The listing builds one solid part. Answer for the finished solid, in the listing's coordinates (mm). A direction names the side the tool comes from. Coordinates: 2 decimals unless noted, no trailing zeros. Write each loop counter-clockwise with the first axis right and the second up, starting at its lowest first coordinate (ties: lowest second). Pieces come first, ordered by that corner, then holes.
Autodesk Inventor part; units mm, degrees
ref_plane "Work Plane1" through (-19.25, -0.5, 9.85) normal (0, 0, 1) x (1, 0, 0)
ref_plane "Work Plane2" through (-19.25, -0.5, 12.85) normal (0, 0, 1) x (1, 0, 0)
ref_plane "Work Plane4" through (19.95, -28.3, 9.85) normal (1, 0, 0) x (0, 0, -1)
ref_plane "Work Plane1" through (-19.25, -0.5, 9.85) normal (0, 0, 1) x (1, 0, 0)
sketch "Sketch1" plane through (-19.25, -0.5, 9.85) normal (0, 0, 1) x (1, 0, 0)
  line L0 (-0.695, -27.8) -> (39.2, -27.8)
  line L1 (39.2, -27.8) -> (39.2, 8.9608)
  line L2 (39.2, 8.9608) -> (-0.695, 8.9608)
  line L3 (-0.695, 8.9608) -> (-0.695, -27.8)
  point P0 (19.25, 0.5)
extrude "Extrusion1" add sketch "Sketch1" along normal blind 3
ref_plane "Work Plane2" through (-19.25, -0.5, 12.85) normal (0, 0, 1) x (1, 0, 0)
sketch "Sketch2" plane through (-19.25, -0.5, 12.85) normal (0, 0, 1) x (1, 0, 0)
  line L0 (39.2, -27.8) -> (39.2, 8.9608)
  line L1 (39.2, -27.8) -> (-0.695, -27.8)
  line L2 (-0.695, -27.8) -> (-0.695, 8.9608)
  line L3 (-0.695, 8.9608) -> (39.2, 8.9608)
  line L4 (39.2, 8.9608) -> (39.2, -27.8)
  point P0 (19.25, 0.5)
  point P1 (39.2, 8.9608)
extrude "Extrusion2" add sketch "Sketch2" along normal blind 5
ref_plane "Work Plane4" through (19.95, -28.3, 9.85) normal (1, 0, 0) x (0, 0, -1)
sketch "Sketch3" plane through (19.95, -28.3, 9.85) normal (1, 0, 0) x (0, 0, -1)
  line L0 (0, 0) -> (0, 36.7608)
  line L1 (0, 0) -> (-8, 0)
  line L2 (0, 36.7608) -> (-2, 36.7608)
  line L3 (-2, 36.7608) -> (-2, 0)
  line L4 (-2, 0) -> (0, 0)
  line L5 (0, 0) -> (0, 36.7608)
  point P0 (9.85, 28.3)
  dimension "d4" = 2
extrude "Extrusion3" cut sketch "Sketch3" against normal blind 50
ref_plane "Work Plane3" through (19.95, -28.3, 17.85) normal (1, 0, 0) x (0, 0, -1)
sketch "Sketch4" plane through (19.95, -28.3, 17.85) normal (1, 0, 0) x (0, 0, -1)
  line L0 (6, 0) -> (0, 0)
  line L1 (6, 36.7608) -> (0, 36.7608)
  line L2 (0, 0) -> (1, 0)
  line L3 (1, 0) -> (1, 36.7608)
  line L4 (1, 36.7608) -> (0, 36.7608)
  line L5 (0, 36.7608) -> (0, 0)
  point P0 (17.85, 28.3)
  point P1 (1, 0)
  dimension "d7" = 1
extrude "Extrusion4" cut sketch "Sketch4" against normal blind 50
ref_plane "Work Plane5" through (19.95, -28.3, 11.85) normal (1, 0, 0) x (0, 0, -1)
sketch "Sketch5" plane through (19.95, -28.3, 11.85) normal (1, 0, 0) x (0, 0, -1)
  line L0 (-5, 36.7608) -> (-5, 0)
  line L1 (0, 0) -> (0, 36.7608)
  line L2 (-5, 36.7608) -> (0, 36.7608)
  line L3 (0, 36.7608) -> (0, 0)
  line L4 (0, 0) -> (-5, 0)
  line L5 (-5, 0) -> (-5, 36.7608)
  point P0 (11.85, 28.3)
extrude "Extrusion5" add sketch "Sketch5" along normal blind 7
ref_plane "Work Plane6" through (-19.945, -28.3, 11.85) normal (0, 0, -1) x (-1, 0, 0)
sketch "Sketch6" plane through (-19.945, -28.3, 11.85) normal (0, 0, -1) x (-1, 0, 0)
  line L0 (-46.895, 0) -> (-46.895, 36.7608)
  line L1 (-46.895, 27.8459) -> (-40.895, 27.8459)
  line L2 (-40.895, 27.8459) -> (-40.895, 11.8459)
  line L3 (-40.895, 11.8459) -> (-46.895, 11.8459)
  line L4 (-46.895, 11.8459) -> (-46.895, 27.8459)
  point P0 (-19.945, 28.3)
  dimension "d12" = 6
  dimension "d13" = 16
extrude "Extrusion6" add sketch "Sketch6" along normal blind 22.875
sketch "Sketch7" plane through (20.95, -0.4541, 11.85) normal (0, 1, 0) x (1, 0, 0)
  arc A0 (5.4164, 8.2173) -> (5.4164, 5.6327) centre (3.7611, 6.925) ccw
  circle A1 centre (3.7611, 6.925) radius 2.5
  arc A2 (5.4164, 18.0673) -> (5.4164, 15.4827) centre (3.7611, 16.775) ccw
  circle A3 centre (3.7611, 16.775) radius 2.5
  point P0 (-20.95, 11.85)
  dimension "d16" = 5
  dimension "d17" = 5
extrude "Extrusion7" cut sketch "Sketch7" against normal blind 22.875
ref_plane "Work Plane7" through (26.95, -28.3, 11.85) normal (1, 0, 0) x (0, 0, -1)
sketch "Sketch8" plane through (26.95, -28.3, 11.85) normal (1, 0, 0) x (0, 0, -1)
  line L0 (0, 11.8459) -> (22.875, 11.8459)
  line L1 (22.875, 27.8459) -> (22.875, 11.8459)
  line L2 (0, 11.8459) -> (22.875, 11.8459)
  line L3 (22.875, 11.8459) -> (22.875, 16.8459)
  line L4 (22.875, 16.8459) -> (0, 16.8459)
  line L5 (0, 16.8459) -> (0, 11.8459)
  point P0 (11.85, 28.3)
  dimension "d20" = 5
extrude "Extrusion8" cut sketch "Sketch8" against normal blind 6.7
ref_plane "Work Plane8" through (-19.945, -28.3, 11.85) normal (-1, 0, 0) x (0, 0, 1)
sketch "Sketch9" plane through (-19.945, -28.3, 11.85) normal (-1, 0, 0) x (0, 0, 1)
  line L0 (0, 36.7608) -> (0, 0)
  line L1 (5, 0) -> (0, 0)
  line L2 (0, 36.7608) -> (5, 36.7608)
  line L3 (5, 36.7608) -> (5, 0)
  line L4 (5, 0) -> (0, 0)
  line L5 (0, 0) -> (0, 36.7608)
  point P0 (-11.85, 28.3)
extrude "Extrusion9" add sketch "Sketch9" along normal blind 7
ref_plane "Work Plane10" through (26.95, -0.4541, 11.85) normal (0, 0, -1) x (-1, 0, 0)
sketch "Sketch11" plane through (26.95, -0.4541, 11.85) normal (0, 0, -1) x (-1, 0, 0)
  line L0 (53.895, -27.8459) -> (53.895, 8.9148)
  line L1 (53.895, 0) -> (47.895, 0)
  line L2 (47.895, 0) -> (47.895, -11)
  line L3 (47.895, -11) -> (53.895, -11)
  line L4 (53.895, -11) -> (53.895, 0)
  point P0 (26.95, 0.4541)
  dimension "d25" = 6
extrude "Extrusion10" add sketch "Sketch11" along normal blind 22.875
sketch "Sketch12" plane through (-26.945, -0.4541, 11.85) normal (0, 1, 0) x (1, 0, 0)
  arc A0 (0.5786, 15.4827) -> (0.5786, 18.0673) centre (2.2339, 16.775) ccw
  circle A1 centre (2.2339, 16.775) radius 2.5
  arc A2 (0.5786, 5.6327) -> (0.5786, 8.2173) centre (2.2339, 6.925) ccw
  circle A3 centre (2.2339, 6.925) radius 2.5
  point P0 (26.945, 11.85)
  dimension "d28" = 5
  dimension "d29" = 5
extrude "Extrusion11" cut sketch "Sketch12" against normal blind 22.875
ref_plane "Work Plane11" through (-26.945, -28.3, 11.85) normal (-1, 0, 0) x (0, 0, 1)
sketch "Sketch13" plane through (-26.945, -28.3, 11.85) normal (-1, 0, 0) x (0, 0, 1)
  line L0 (0, 16.8459) -> (0, 27.8459)
  line L1 (5, 36.7608) -> (0, 36.7608)
  line L2 (0, 27.8459) -> (5, 27.8459)
  line L3 (5, 27.8459) -> (5, 36.7608)
  line L4 (5, 36.7608) -> (0, 36.7608)
  line L5 (0, 36.7608) -> (0, 27.8459)
  point P0 (-11.85, 28.3)
extrude "Extrusion12" cut sketch "Sketch13" against normal blind 67.325
ref_plane "Work Plane9" through (26.95, -28.3, 11.85) normal (0, -1, 0) x (1, 0, 0)
sketch "Sketch14" plane through (26.95, -28.3, 11.85) normal (0, -1, 0) x (1, 0, 0)
  line L0 (0, 5) -> (0, 0)
  line L1 (0, 5) -> (-53.895, 5)
  line L2 (0, 0) -> (-53.895, 0)
  line L3 (-53.895, 0) -> (-53.895, 5)
  line L4 (-53.895, 5) -> (0, 5)
  line L5 (0, 5) -> (0, 0)
  point P0 (-26.95, -11.85)
extrude "Extrusion13" add sketch "Sketch14" along normal blind 5
ref_plane "Work Plane12" through (26.95, -11.4541, 11.85) normal (0, 0, -1) x (-1, 0, 0)
sketch "Sketch15" plane through (26.95, -11.4541, 11.85) normal (0, 0, -1) x (-1, 0, 0)
  line L0 (53.895, -21.8459) -> (0, -21.8459)
  line L1 (53.895, 11) -> (53.895, -21.8459)
  line L2 (0, -21.8459) -> (53.895, -21.8459)
  line L3 (53.895, -21.8459) -> (53.895, -17.8459)
  line L4 (53.895, -17.8459) -> (0, -17.8459)
  line L5 (0, -17.8459) -> (0, -21.8459)
  point P0 (26.95, 11.4541)
  dimension "d36" = 4
extrude "Extrusion14" add sketch "Sketch15" along normal blind 22.4625
ref_plane "Work Plane13" through (-26.945, -29.3, 11.85) normal (0, 1, 0) x (1, 0, 0)
sketch "Sketch16" plane through (-26.945, -29.3, 11.85) normal (0, 1, 0) x (1, 0, 0)
  line L0 (53.895, 0) -> (53.895, 22.4625)
  line L1 (0, 0) -> (0, 22.4625)
  line L2 (53.895, 0) -> (0, 0)
  line L3 (0, 0) -> (0, 1)
  line L4 (0, 1) -> (53.895, 1)
  line L5 (53.895, 1) -> (53.895, 0)
  point P0 (26.945, 11.85)
  point P1 (53.895, 1)
  dimension "d39" = 1
extrude "Extrusion15" add sketch "Sketch16" along normal blind 30
ref_plane "Work Plane14" through (26.95, -28.3, 11.85) normal (1, 0, 0) x (0, 0, -1)
sketch "Sketch17" plane through (26.95, -28.3, 11.85) normal (1, 0, 0) x (0, 0, -1)
  line L0 (0, 29) -> (1, 29)
  line L1 (5.8126, 27.8459) -> (1, 27.8459)
  line L2 (0, 29) -> (1, 29)
  line L3 (1, 29) -> (1, 27.8459)
  line L4 (1, 27.8459) -> (0, 27.8459)
  line L5 (0, 27.8459) -> (0, 29)
  point P0 (11.85, 28.3)
extrude "Extrusion16" cut sketch "Sketch17" against normal blind 100
sketch "Sketch19" plane through (26.95, -33.3, 11.85) normal (0, -1, 0) x (1, 0, 0)
  circle A0 centre (-16.85, -11.85) radius 5
  circle A1 centre (-16.85, -11.85) radius 1.5
  point P0 (-26.95, -11.85)
  dimension "d47" = 10
  dimension "d50" = 3
extrude "Extrusion20" cut sketch "Sketch19" against normal blind 10 contours A1
sketch "Sketch20" plane through (26.95, -33.3, 11.85) normal (0, -1, 0) x (1, 0, 0)
  line L0 (-53.895, -22.4625) -> (0, -22.4625)
  line L1 (-53.895, 5) -> (-53.895, -22.4625)
  line L2 (0, -22.4625) -> (-53.895, -22.4625)
  line L3 (-53.895, -22.4625) -> (-53.895, 5)
  line L4 (-53.895, 5) -> (0, 5)
  line L5 (0, 5) -> (0, -22.4625)
  point P0 (-26.95, -11.85)
extrude "Extrusion21" add sketch "Sketch20" along normal blind 2
sketch "Sketch21" plane through (-26.945, -29.3, -10.6125) normal (0, 1, 0) x (1, 0, 0)
  circle A0 centre (37.045, -10.6125) radius 1.5
  circle A1 centre (37.045, -10.6125) radius 1.5
  point P0 (26.945, -10.6125)
extrude "Extrusion22" cut sketch "Sketch21" against normal blind 10
sketch "Sketch22" plane through (-26.945, -29.3, -10.6125) normal (0, 1, 0) x (1, 0, 0)
  circle A0 centre (37.045, -10.6125) radius 1.5
  circle A1 centre (37.045, -10.6125) radius 2.5
  point P0 (26.945, -10.6125)
  dimension "d59" = 5
extrude "Extrusion23" cut sketch "Sketch22" against normal blind 2
sketch "Sketch23" plane through (-19.945, -28.3, -11.025) normal (0, 0, -1) x (-1, 0, 0)
  line L0 (-46.895, 27.8459) -> (-46.895, 16.8459)
  line L1 (-46.895, 27.8459) -> (-48.895, 27.8459)
  line L2 (-48.895, 27.8459) -> (-48.895, 16.8459)
  line L3 (-48.895, 16.8459) -> (-46.895, 16.8459)
  line L4 (-46.895, 16.8459) -> (-46.895, 27.8459)
  line L5 (7, 16.8459) -> (7, 27.8459)
  line L6 (7, 27.8459) -> (9, 27.8459)
  line L7 (9, 27.8459) -> (9, 16.8459)
  line L8 (9, 16.8459) -> (7, 16.8459)
  line L9 (7, 16.8459) -> (7, 27.8459)
  point P0 (-19.945, 28.3)
  dimension "d62" = 2
  dimension "d63" = 2
extrude "Extrusion24" add sketch "Sketch23" against normal up to surface (27.875 mm away)
sketch "Sketch24" plane through (-20.945, -0.4541, 10.85) normal (0, 1, 0) x (1, 0, 0)
  arc A0 (47.895, 7.0374) -> (47.895, 4.8126) centre (45.6561, 5.925) ccw
  circle A1 centre (45.6561, 5.925) radius 1.6
  arc A2 (47.895, 16.8874) -> (47.895, 14.6626) centre (45.6561, 15.775) ccw
  circle A3 centre (45.6561, 15.775) radius 1.6
  circle A4 centre (45.6561, 5.925) radius 2.5
  circle A5 centre (45.6561, 15.775) radius 2.5
  point P0 (20.945, 10.85)
  point P1 (47.895, 4.8126)
  dimension "d66" = 3.2
  dimension "d67" = 3.2
extrude "Extrusion25" add sketch "Sketch24" against normal up to surface (11 mm away)
sketch "Sketch25" plane through (-20.945, -0.4541, 10.85) normal (0, 1, 0) x (1, 0, 0)
  arc A0 (-6, 4.8025) -> (-6, 7.0475) centre (-3.7661, 5.925) ccw
  circle A1 centre (-3.7661, 5.925) radius 1.6
  arc A2 (-6, 14.6525) -> (-6, 16.8975) centre (-3.7661, 15.775) ccw
  circle A3 centre (-3.7661, 15.775) radius 1.6
  circle A4 centre (-3.7661, 15.775) radius 2.5
  circle A5 centre (-3.7661, 5.925) radius 2.5
  point P0 (20.945, 10.85)
  point P1 (-6, 7.0475)
  dimension "d70" = 3.2
  dimension "d71" = 3.2
  dimension "d72" = 5
  dimension "d73" = 5
extrude "Extrusion26" add sketch "Sketch25" against normal up to surface (11 mm away)
sketch "Sketch26" plane through (-26.945, -35.3, 16.85) normal (0, 0, 1) x (1, 0, 0)
  line L0 (55.895, 34.8459) -> (-2, 34.8459)
  line L1 (53.895, 23.8459) -> (55.895, 23.8459)
  line L2 (-2, 34.8459) -> (55.895, 34.8459)
  line L3 (55.895, 34.8459) -> (55.895, 23.8459)
  line L4 (55.895, 23.8459) -> (-2, 23.8459)
  line L5 (-2, 23.8459) -> (-2, 34.8459)
  point P0 (26.945, 35.3)
extrude "Extrusion27" add sketch "Sketch26" along normal blind 20
sketch "Sketch27" plane through (-20.945, -0.4541, 10.85) normal (0, 1, 0) x (1, 0, 0)
  line L0 (49.895, 21.875) -> (49.895, -26)
  line L1 (49.895, -26) -> (49.895, -16)
  line L2 (49.895, -16) -> (-8, -16)
  line L3 (-8, 21.875) -> (-8, -26)
  line L4 (49.895, -16) -> (31.895, -16)
  line L5 (-8, -16) -> (10, -16)
  circle A0 centre (31.895, -16) radius 5
  circle A1 centre (10, -16) radius 5
  point P0 (20.945, 10.85)
  dimension "d78" = 10
  dimension "d79" = 18
  dimension "d80" = 18
  dimension "d81" = 10
  dimension "d82" = 10
hole "Hole1" at (-10.945, -0.4541, 26.85) at (10.95, -0.4541, 26.85) direction (0, -1, 0) diameter 5 end through all countersink diameter 10 countersink angle 90
sketch "Sketch28" plane through (-26.945, -29.3, -10.6125) normal (0, 1, 0) x (1, 0, 0)
  circle A0 centre (37.045, -10.6125) radius 2.5
  line L0 (37.045, -10.6125) -> (53.895, -10.6125)
  line L1 (53.895, 0) -> (53.895, -27.4625)
  line L2 (0, -27.4625) -> (0, 0)
  line L3 (0, -10.6125) -> (16.85, -10.6125)
  line L4 (0, -10.6125) -> (16.85, -10.6125) construction
  line L5 (16.85, -10.6125) -> (37.045, -10.6125)
  circle A1 centre (16.85, -10.6125) radius 1.5
  point P0 (26.945, -10.6125)
  dimension "d90" = 16.85
  dimension "d91" = 0
  dimension "d92" = 3
extrude "Extrusion28" cut sketch "Sketch28" against normal blind 10 contours A1 L3 L5 | L5 L3 A1
sketch "Sketch29" plane through (-26.945, -29.3, -10.6125) normal (0, 1, 0) x (1, 0, 0)
  circle A0 centre (16.85, -10.6125) radius 1.5
  circle A1 centre (16.85, -10.6125) radius 2.5
  point P0 (26.945, -10.6125)
  dimension "d95" = 5
extrude "Extrusion29" cut sketch "Sketch29" against normal up to surface (2 mm away) contours A0 | A1
sketch "Sketch30" plane through (-26.945, -29.3, -10.6125) normal (0, 1, 0) x (1, 0, 0)
  circle A0 centre (37.045, -10.6125) radius 2.5
  circle A1 centre (37.045, -10.6125) radius 2.5
  point P0 (26.945, -10.6125)
extrude "Extrusion30" add sketch "Sketch30" against normal up to surface (6 mm away)
properties part number "woodHold" material "钢"
Q1. Determine the mould class of faces 4 (the face through (-11.594, -33.272, -0.066)), 5 (the face through (0, -6, 36.85)), 6 (the face through (26.95, -31, 9)) for opening direction X: released by +X, released by -X, zero draft, split by the parting line, or undercut.
Answers below:
face 4: undercut
face 5: zero draft
face 6: released by +X
Q2. Given pin 1 (1.8 mm diameter, centred on x = -10.095, z = 0, fed in from +Y); pin 2 (1 mm diameter, centred on x = 1, y = -28.5, fed in from +Z); pin 3 (1.5 mm diameter, centred on x = -11, z = 0, fed in from +Y); pin 4 (14.5 mm diameter, centred on x = 4.5, y = -16, fed in from -Z), each flat-ended and moving along its own axis, determine where each tip first touches the part or whether it passes through.
Answers below:
pin 1: passes through
pin 2: stops at z = 16.85
pin 3: stops at y = -31.3
pin 4: stops at z = 10.85
Q3. The part is cut by section A-A, the plane z = 0. Write down the section's boundary in (x, y) (3 decimals).
Answers below:
outline: (-28.945, -11.454) - (-20.945, -11.454) - (-20.945, -0.454) - (-28.945, -0.454) - close; (-26.945, -35.3) - (-11.595, -35.3) - (-11.595, -31.3) - (-12.595, -31.3) - (-12.595, -29.3) - (-26.945, -29.3) - close; (-8.595, -35.3) - (26.95, -35.3) - (26.95, -29.3) - (-7.595, -29.3) - (-7.595, -31.3) - (-8.595, -31.3) - close; (20.95, -11.454) - (28.95, -11.454) - (28.95, -0.454) - (20.95, -0.454) - close
Q4. Which of the six approach directions +Z, -Z, +X, -X, +Y, -Y give full straight-line access (tool end or side, diameter ignored) to faces 1 (the face through (0, -29.3, 0)), 2 (the face through (0, -23, 16.85)), 3 (the face through (23.532, -5.877, 3.844))?
Answers below:
face 1: -Z, +X, -X
face 2: +Z, +X, -X, -Y
face 3: +Y
Q5. The part is cut by section D-D, the plane x = 1. Write down the section's boundary in (y, z), then the cut area to 3 significant figures.
Answers below:
outline: (-35.3, -10.61) - (-29.3, -10.61) - (-29.3, 10.85) - (-0.45, 10.85) - (-0.45, 36.85) - (-11.45, 36.85) - (-11.45, 16.85) - (-35.3, 16.85) - close
area: 558 mm2
Q6. The part is cut by section C-C, the plane z = 26.85. Write down the section's boundary in (x, y) (3 decimals), then the cut area to 3 significant figures.
Answers below:
outline: (-28.945, -11.454) - (-13.445, -11.454) - (-13.445, -2.954) - (-15.945, -0.454) - (-28.945, -0.454) - close; (-8.445, -11.454) - (8.45, -11.454) - (8.45, -2.954) - (5.95, -0.454) - (-5.945, -0.454) - (-8.445, -2.954) - close; (13.45, -11.454) - (28.95, -11.454) - (28.95, -0.454) - (15.95, -0.454) - (13.45, -2.954) - close
area: 514 mm2
Q7. The part is cut by section B-B, the plane x = 10.95. Write down the section's boundary in (y, z), then the cut area to 3 significant figures.
Answers below:
outline: (-35.3, -10.61) - (-29.3, -10.61) - (-29.3, 10.85) - (-0.45, 10.85) - (-0.45, 21.85) - (-2.95, 24.35) - (-11.45, 24.35) - (-11.45, 16.85) - (-35.3, 16.85) - close; (-11.45, 29.35) - (-2.95, 29.35) - (-0.45, 31.85) - (-0.45, 36.85) - (-11.45, 36.85) - close
area: 497 mm2
Q8. Find the intervals of material crossed by probe 1 along X at (y, z) = (-10.5, 5) (3 decimals); probe 2 along X at (y, z) = (-33, 0) (3 decimals); probe 3 along Y at (x, z) = (-26, 3), in increasing order.
Answers below:
probe 1: x = -28.945 to -26.309, -23.113 to -20.945, 20.95 to 23.113, 26.309 to 28.95
probe 2: x = -26.945 to -11.595, -8.595 to 26.95
probe 3: y = -35.3 to -29.3, -11.45 to -0.45
